Source: three-view drawing plus pictorial views. Frame: mm from the lowest corner of the part. A direction names the side the tool comes from. Give positions to 0.01 mm unless a question says otherwise; leave off trailing zeros. Write each loop counter-clockwise with the first axis right and the second up, starting at its lowest first coordinate (ties: lowest second). Pieces come first, ordered by that corner, then holes.
Q1. Cut plane A-A on x = 8. Return the cut outline in (y, z).
Q2. Cut plane C-C on x = 30.5. Return the cut outline in (y, z).
Q3. Cut plane B-B on z = 6. Return the cut outline in (x, y).
Q4. Reachability of the marked faces 1, 2 and 3 from +Z, -Z, +X, -X, +Y, -Y: full face, straight path, thin tool, end or side. Return the list, or none.
Q5. Cut plane D-D on y = 3. Return the cut outline in (x, z), plus the area to 4 significant figures.
Q6. Line query: L1, parallel to X at y = 13, z = 4.25; L2, parallel to Y at x = 30.5, z = 4.5; L3, parallel to X at y = 14.5, z = 5. Output: solid intervals per line, ascending.
Q7. Draft query along Y for the marked faces 4, 5 and 6. Return one class per face: pulls with the +Y half, pulls with the -Y half, needs draft (parallel to the pull), parting line crosses it, or undercut.
Q8. Pin query (flat end, axial travel): pin 1 (1.8 mm diameter, centred on x = 2.5, z = 4.5, fed in from -Y); pin 2 (1 mm diameter, centred on y = 7.5, z = 3, fed in from +X). Return the tip coordinate at first contact, or that it passes through.
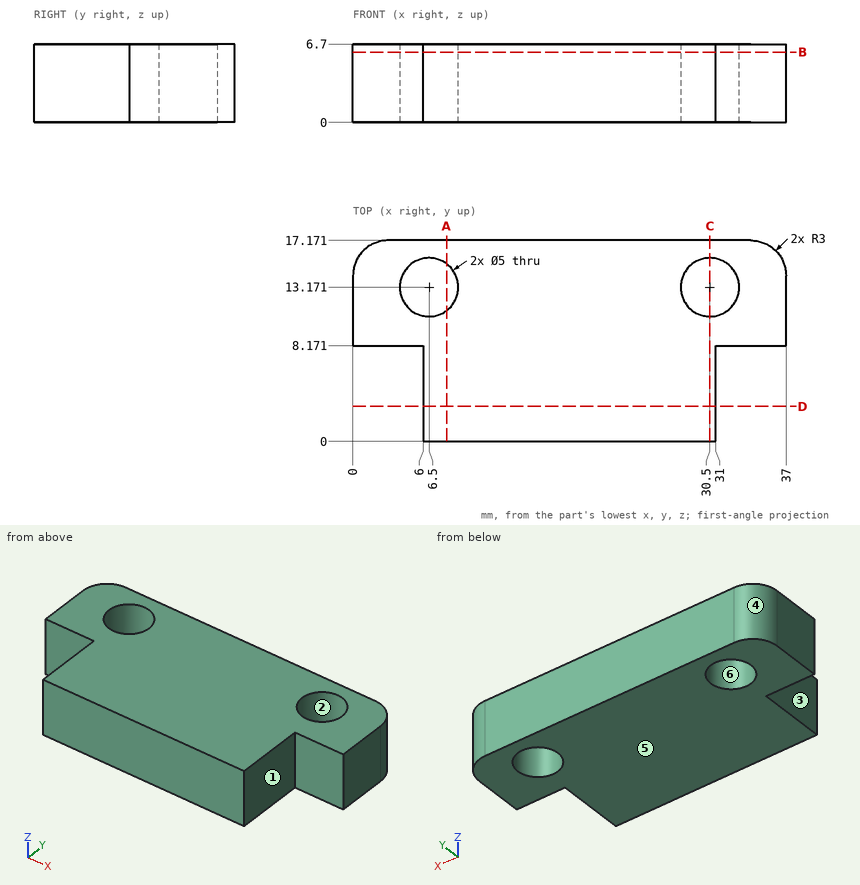
Data:
1. outline: (0, 0) - (11.17, 0) - (11.17, 6.7) - (0, 6.7) - close; (15.17, 0) - (17.17, 0) - (17.17, 6.7) - (15.17, 6.7) - close
2. outline: (0, 0) - (10.67, 0) - (10.67, 6.7) - (0, 6.7) - close; (15.67, 0) - (17.17, 0) - (17.17, 6.7) - (15.67, 6.7) - close
3. outline: (0, 8.17) - (6, 8.17) - (6, 0) - (31, 0) - (31, 8.17) - (37, 8.17) - (37, 14.17) arc R3 ccw to (34, 17.17) - (3, 17.17) arc R3 ccw to (0, 14.17) - close; hole circle Ø5 at (6.5, 13.17); hole circle Ø5 at (30.5, 13.17)
4. face 1: +Z, -Z, +X, -Y
4. face 2: +Z, -Z
4. face 3: +Z, -Z, -X, -Y
5. outline: (6, 0) - (31, 0) - (31, 6.7) - (6, 6.7) - close
5. area: 167.5 mm2
6. L1: x = 0 to 4.01, 8.99 to 28.01, 32.99 to 37
6. L2: y = 0 to 10.67, 15.67 to 17.17
6. L3: x = 0.02 to 4.38, 8.62 to 28.38, 32.62 to 36.98
7. face 4: pulls with the +Y half
7. face 5: needs draft
7. face 6: undercut
8. pin 1: stops at y = 8.17
8. pin 2: stops at x = 31
